Part model, mm, in its own coordinate system. Face numbers are marked on the shaded views. A direction names the side the tool comes from. Round coordinates to 2 decimals unless told otherwise and drop trailing zeros. Loops run counter-clockwise (first coordinate to the right, second up) from the corner with the lowest first, then second, coordinate; pieces in that order, holes last. Notation, with made-up numbers: M 54.25,39.25 L 110.25,39.25 A25 cw 110.25,69.25 Z; hole C -18,-27.75 d1. An arc over 180 degrees is marked long. Write each question's results on one line, items separated by ' | '.
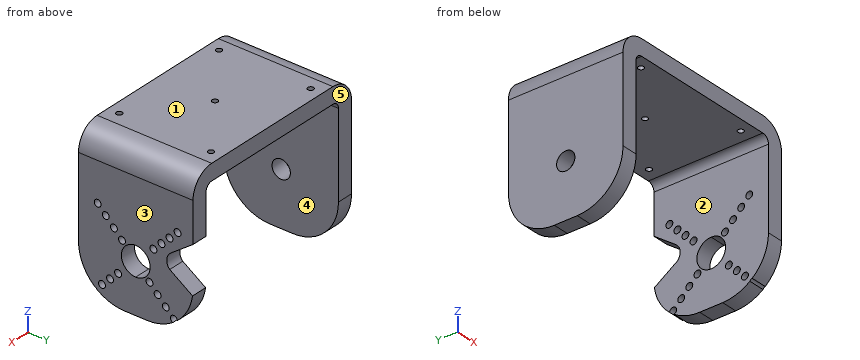
from build123d import *

# Parameters (mm, degrees)
BOSS_EXTRUDE1_DEPTH     = 50
FILLET2_R               = 20
SKETCH6_R               = 1.5
CUT_EXTRUDE2_DEPTH      = 28.4
CUT_EXTRUDE3_DEPTH      = 136.4
CUT_EXTRUDE4_DEPTH      = 120.503043838
CUT_EXTRUDE4_DEPTH_BACK = 26.4
SKETCH8_R               = 1.25
CUT_EXTRUDE5_DEPTH      = 100


with BuildPart() as part:
    # Sketch1 → Boss-Extrude1 (new body)
    with BuildSketch(Plane(origin=(0, 0, 0), x_dir=(1, 0, 0), z_dir=(0, 1, 0))):
        with BuildLine():
            Line((-56.375697839, 67.497981352), (-56.375697839, 10.497981352))
            ThreePointArc((-56.375697839, 10.497981352), (-53.44676565, 3.42691354), (-46.375697839, 0.497981352))
            Line((-46.375697839, 0.497981352), (18.624302161, 0.497981352))
            ThreePointArc((18.624302161, 0.497981352), (25.695369973, 3.42691354), (28.624302161, 10.497981352))
            Line((28.624302161, 10.497981352), (28.624302161, 65.497981352))
            Line((28.624302161, 65.497981352), (21.624302161, 65.497981352))
            Line((21.624302161, 65.497981352), (21.624302161, 10.497981352))
            ThreePointArc((21.624302161, 10.497981352), (20.745622505, 8.376661008), (18.624302161, 7.497981352))
            Line((18.624302161, 7.497981352), (-46.375697839, 7.497981352))
            ThreePointArc((-46.375697839, 7.497981352), (-48.497018182, 8.376661008), (-49.375697839, 10.497981352))
            Line((-49.375697839, 10.497981352), (-49.375697839, 67.497981352))
            Line((-49.375697839, 67.497981352), (-56.375697839, 67.497981352))
        make_face()
    extrude(amount=BOSS_EXTRUDE1_DEPTH)

    # Fillet2
    fillet2_edges = [part.edges().sort_by_distance(p)[0] for p in [
        (25.124302161, 0, -65.497981352),
        (-52.875697839, 0, -67.497981352),
        (25.124302161, 50, -65.497981352),
        (-52.875697839, 50, -67.497981352),
    ]]
    fillet(fillet2_edges, radius=FILLET2_R)

    # Sketch6 → Cut-Extrude2 (cut)
    with BuildSketch(Plane(origin=(28.624302161, 0, 0), x_dir=(0, 0, -1), z_dir=(1, 0, 0))):
        with BuildLine():
            ThreePointArc((39.997981352, 25), (43.997981352, 21), (47.997981352, 25))
            Line((47.997981352, 25), (39.997981352, 25))
        make_face()
        with BuildLine():
            Line((39.997981352, 25), (47.997981352, 25))
            ThreePointArc((47.997981352, 25), (43.997981352, 29), (39.997981352, 25))
        make_face()
        with BuildLine():
            ThreePointArc((37.736343923, 25), (43.997981352, 18.738362572), (50.25961878, 25))
            Line((50.25961878, 25), (47.997981352, 25))
            ThreePointArc((47.997981352, 25), (43.997981352, 21), (39.997981352, 25))
            Line((39.997981352, 25), (37.736343923, 25))
        make_face()
        with BuildLine():
            Line((47.997981352, 25), (50.25961878, 25))
            ThreePointArc((50.25961878, 25), (43.997981352, 31.261637428), (37.736343923, 25))
            Line((37.736343923, 25), (39.997981352, 25))
            ThreePointArc((39.997981352, 25), (43.997981352, 29), (47.997981352, 25))
        make_face()
        with Locations((36.290517437, 32.707463915)):
            Circle(SKETCH6_R)
        with Locations((32.776196734, 36.221784617)):
            Circle(SKETCH6_R)
        with Locations((29.254804964, 39.743176388)):
            Circle(SKETCH6_R)
        with Locations((25.754626397, 43.243354955)):
            Circle(SKETCH6_R)
        with Locations((50.008388992, 31.01040764)):
            Circle(SKETCH6_R)
        with Locations((53.543922898, 34.545941546)):
            Circle(SKETCH6_R)
        with Locations((57.079456803, 38.081475452)):
            Circle(SKETCH6_R)
        with Locations((60.614990709, 41.617009358)):
            Circle(SKETCH6_R)
        with Locations((51.705445266, 17.292536085)):
            Circle(SKETCH6_R)
        with Locations((55.219765969, 13.778215383)):
            Circle(SKETCH6_R)
        with Locations((58.741157739, 10.256823612)):
            Circle(SKETCH6_R)
        with Locations((62.241336306, 6.756645045)):
            Circle(SKETCH6_R)
        with Locations((37.987573711, 18.98959236)):
            Circle(SKETCH6_R)
        with Locations((34.452039805, 15.454058454)):
            Circle(SKETCH6_R)
        with Locations((30.9165059, 11.918524548)):
            Circle(SKETCH6_R)
        with Locations((27.380971994, 8.382990642)):
            Circle(SKETCH6_R)
    extrude(amount=-CUT_EXTRUDE2_DEPTH, mode=Mode.SUBTRACT)

    # Sketch6<3> → Cut-Extrude3 (cut)
    with BuildSketch(Plane(origin=(28.624302161, 0, 0), x_dir=(0, 0, -1), z_dir=(1, 0, 0))):
        with BuildLine():
            ThreePointArc((39.997981352, 25), (43.997981352, 21), (47.997981352, 25))
            Line((47.997981352, 25), (39.997981352, 25))
        make_face()
        with BuildLine():
            Line((39.997981352, 25), (47.997981352, 25))
            ThreePointArc((47.997981352, 25), (43.997981352, 29), (39.997981352, 25))
        make_face()
    extrude(amount=-CUT_EXTRUDE3_DEPTH, mode=Mode.SUBTRACT)

    # Sketch7 → Cut-Extrude4 (cut, two sides: drawn at the far end of the back side and taken through both)
    with BuildSketch(Plane(origin=(28.624302161, 0, 0), x_dir=(0, 0, -1), z_dir=(1, 0, 0)).offset(-CUT_EXTRUDE4_DEPTH_BACK)):
        with BuildLine():
            Line((-59.021683843, 169.857328721), (27.901409821, 50))
            Line((27.901409821, 50), (34.889942889, 40.363586132))
            ThreePointArc((34.889942889, 40.363586132), (38.136702541, 38.542544558), (41.629478365, 39.830239282))
            Line((41.629478365, 39.830239282), (48.296449702, 49.803246574))
            Line((48.296449702, 49.803246574), (130.580983454, 172.89125966))
            Line((130.580983454, 172.89125966), (125.843258674, 468.970924285))
            Line((125.843258674, 468.970924285), (-63.759408622, 465.936993346))
            Line((-63.759408622, 465.936993346), (-59.021683843, 169.857328721))
        make_face()
    extrude(amount=CUT_EXTRUDE4_DEPTH + CUT_EXTRUDE4_DEPTH_BACK, mode=Mode.SUBTRACT)

    # Sketch8 → Cut-Extrude5 (cut)
    with BuildSketch(Plane.XY.offset(-0.497981352)):
        with Locations((-40.625697839, 45)):
            Circle(SKETCH8_R)
        with Locations((12.874302161, 45)):
            Circle(SKETCH8_R)
        with Locations((-13.875697839, 25)):
            Circle(SKETCH8_R)
        with Locations((-40.625697839, 5)):
            Circle(SKETCH8_R)
        with Locations((12.874302161, 5)):
            Circle(SKETCH8_R)
    extrude(amount=-CUT_EXTRUDE5_DEPTH, mode=Mode.SUBTRACT)


solid = part.part
Item 1: Drop flat-ended pins along their axis: P1, Ø2, axis at x = 23.5, y = 24, coming from the -Z side; P2, Ø5, axis at y = 10.26, z = -58.74, coming from the +X side; P3, Ø6, axis at x = 11.5, y = 31.5, coming from the -Z side; P4, Ø1.8, axis at y = 38.08, z = -57.08, coming from the +X side. Give the stop position or say it passes through.
Filled sheet:
P1: z = -65.5 | P2: x = 28.62 | P3: z = -7.5 | P4: x = -49.38
Item 2: Which spindle directions (+Z, -Z, +X, -X, +Y, -Y) get a long thin tool onto all of the face, cutting with end or side? Do the marked faces 4 and 5. Say none if no direction does.
Filled sheet:
face 4: -Z, +Y, -Y | face 5: +Z, -Z, +X, -X, +Y
Item 3: Two-plate mould, pull along X, no slides. Class the marked faces 1, 2 and 3: +X half, -X half, draft (parallel to the pull), parting line (faces both ways), or undercut.
Filled sheet:
face 1: draft | face 2: undercut | face 3: +X half
Item 4: Band-saw the part on C-C on x = 6.5. Give the cut face in (y, z), and give its area (3 significant figures).
Filled sheet:
outline: M 0,-7.5 L 50,-7.5 L 50,-0.5 L 0,-0.5 Z | area: 350 mm^2
Item 5: Wall check: L1, parallel to X at y = 29, z = -62.5; L2, parallel to Z at x = -1, y = 25; L3, parallel to Y at x = -50, z = -42. Give the ranges that are in metal, low to high.
Filled sheet:
L1: -56.38 to -49.38, 21.62 to 28.62 | L2: -7.5 to -0.5 | L3: 0 to 21.53, 28.47 to 50
Item 6: Band-saw the part on B-B on y = 5. Give the cut face in (x, z), and give its area (3 significant figures).
Filled sheet:
outline: M -56.38,-60.73 L -49.38,-60.73 L -49.38,-10.5 A3 cw -46.38,-7.5 L -41.88,-7.5 L -41.88,-0.5 L -46.38,-0.5 A10 ccw -56.38,-10.5 Z; M -39.38,-7.5 L 11.62,-7.5 L 11.62,-0.5 L -39.38,-0.5 Z; M 14.12,-7.5 L 18.62,-7.5 A3 cw 21.62,-10.5 L 21.62,-58.73 L 28.62,-58.73 L 28.62,-10.5 A10 ccw 18.62,-0.5 L 14.12,-0.5 Z | area: 1,250 mm^2
Item 7: Band-saw the part on A-A on z = -12. Give the cut face in (x, y).
Filled sheet:
outline: M -56.38,0 L -49.38,0 L -49.38,50 L -56.38,50 Z; M 21.62,0 L 28.62,0 L 28.62,50 L 21.62,50 Z
